Here's how the part is built. I have some questions about the finished solid (model axes, mm). Give positions to 0.01 mm unless a question says otherwise; leave off trailing zeros. Loops run counter-clockwise (first coordinate to the right, second up) from the corner with the lowest first, then second, coordinate; pieces in that order, holes last. Notation, with made-up numbers: (7.5, 49) - (37.5, 49) arc R16 ccw to (37.5, 76) - close; hole circle Ø1 at (16, 29.5). An arc over 180 degrees is marked (long way). Use a Markdown table: item, result.
from build123d import *

# Parameters (mm, degrees)
SKETCH1_W                 = 6.35
SKETCH1_H                 = 15.875
EXTRUDE1_DEPTH            = 38.1
M6X1_0_TAPPED_HOLE1_D     = 5
M6X1_0_TAPPED_HOLE1_DEPTH = 6.35


with BuildPart() as part:
    # Sketch1 → Extrude1 (new body, symmetric)
    with BuildSketch(Plane.XY):
        Rectangle(SKETCH1_W, SKETCH1_H)
    extrude(amount=EXTRUDE1_DEPTH, both=True)

    # M6x1.0 Tapped Hole1
    with Locations(Plane(origin=(3.175, 0, 0), x_dir=(0, 0, -1), z_dir=(1, 0, 0))):
        with Locations((-19.05, 0), (19.05, 0)):
            Hole(M6X1_0_TAPPED_HOLE1_D / 2, depth=M6X1_0_TAPPED_HOLE1_DEPTH)


solid = part.part
(1) Suppose I cut it at C-C on x = 2.5. Write out the boundary of the cut face in (y, z).
A:
| item | result |
|---|---|
| outline | (-7.94, -38.1) - (7.94, -38.1) - (7.94, 38.1) - (-7.94, 38.1) - close; hole circle Ø5 at (0, -19.05); hole circle Ø5 at (0, 19.05) |
(2) If I drill on line 1 (Z direction, x = -0.75, y = 0.5); line 2 (Y direction, x = 0.75, z = -19.05); line 3 (Z direction, x = -0.5, y = -2.25), over which ranges is the centre line in solid material (lowest first)?
A:
| item | result |
|---|---|
| line 1 | -38.1 to -21.5, -16.6 to 16.6, 21.5 to 38.1 |
| line 2 | -7.94 to -2.5, 2.5 to 7.94 |
| line 3 | -38.1 to -20.14, -17.96 to 17.96, 20.14 to 38.1 |
(3) Suppose I cut it at B-B on y = 0. Write out the boundary of the cut face in (x, z) (3 decimals).
A:
| item | result |
|---|---|
| outline | (-3.175, -38.1) - (3.175, -38.1) - (3.175, -21.55) - (-3.175, -21.55) - close; (-3.175, -16.55) - (3.175, -16.55) - (3.175, 16.55) - (-3.175, 16.55) - close; (-3.175, 21.55) - (3.175, 21.55) - (3.175, 38.1) - (-3.175, 38.1) - close |
(4) Will this pin go through, and if not, where does the flat tip stop? pin 1 (6 mm diameter, centred on y = 0, z = -19.05, fed in from +X) (3 decimals).
A:
| item | result |
|---|---|
| pin 1 | x = 3.175 |
(5) Suppose I cut it at A-A on z = -19.05. Write out the boundary of the cut face in (x, y) (1 decimal).
A:
| item | result |
|---|---|
| outline | (-3.2, -7.9) - (3.2, -7.9) - (3.2, -2.5) - (-3.2, -2.5) - close; (-3.2, 2.5) - (3.2, 2.5) - (3.2, 7.9) - (-3.2, 7.9) - close |
(6) We'd pull the mould along Y, two halves only. Please class faces 1 (the face through (-0.04, -2.44, -19.59)), 2 (the face through (0, 7.938, 1)), 3 (the face through (3.175, 0, 1)): pulls with the +Y half, pulls with the -Y half, needs draft (parallel to the pull), parting line crosses it, or undercut.
A:
| item | result |
|---|---|
| face 1 | undercut |
| face 2 | pulls with the +Y half |
| face 3 | needs draft |
